Geometry check sheet. Reference: the model listing, model coordinates, mm. Face numbers are marked on the shaded views. A direction names the side the tool comes from. Give positions to 0.01 mm unless a question says otherwise; leave off trailing zeros. Loops run counter-clockwise (first coordinate to the right, second up) from the corner with the lowest first, then second, coordinate; pieces in that order, holes last. Notation, with made-up numbers: (-4.5, 50.25) -> (40.5, 50.25) arc R16 ccw to (40.5, 56.25) -> close; hole circle Ø2 at (-16, -13.5). An arc over 180 degrees is marked (long way). One line per question, with ' | ' between items.
from build123d import *

# Parameters (mm, degrees)
F0_W     = 80
F0_H     = 40
F1_DEPTH = 5
F2_W     = 66
F2_H     = 28
F2_W_2   = 60
F2_H_2   = 22
F3_DEPTH = 15
F4_R     = 2
F5_SIZE  = 1


with BuildPart() as f1:
    # F0 (on Top) → F1 (new body)
    with BuildSketch(Plane.XY):
        Rectangle(F0_W, F0_H)
    extrude(amount=F1_DEPTH)

    # F2 (on face) → F3 (join)
    with BuildSketch(Plane.XY.offset(5)):
        Rectangle(F2_W, F2_H)
        Rectangle(F2_W_2, F2_H_2, mode=Mode.SUBTRACT)
    extrude(amount=F3_DEPTH)

    # F4
    f4_edges = [f1.edges().sort_by_distance(p)[0] for p in [
        (0, -20, 0),
        (-40, 0, 0),
        (0, 20, 0),
        (40, 0, 0),
    ]]
    fillet(f4_edges, radius=F4_R)

    # F5
    f5_edges = [f1.edges().sort_by_distance(p)[0] for p in [
        (-33, -14, 12.5),
        (-33, 14, 12.5),
        (33, -14, 12.5),
        (33, 14, 12.5),
    ]]
    chamfer(f5_edges, length=F5_SIZE)


solid = f1.part
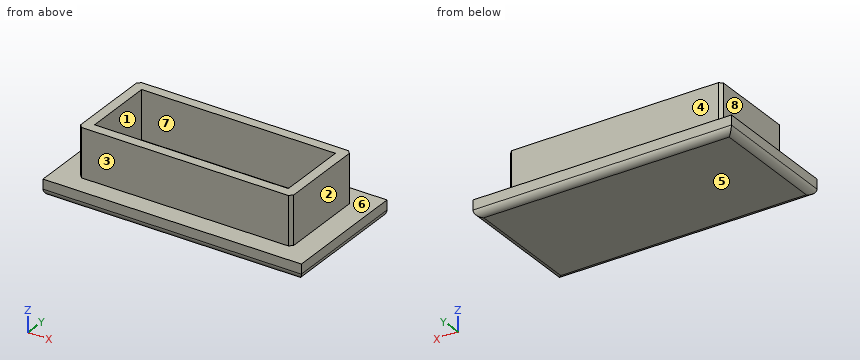
Item 1: Sectioned sample at B-B (y = 0). Record the cut outline in (x, z).
Result:
outline: (-40, 2) arc R2 ccw to (-38, 0) -> (38, 0) arc R2 ccw to (40, 2) -> (40, 5) -> (33, 5) -> (33, 20) -> (30, 20) -> (30, 5) -> (-30, 5) -> (-30, 20) -> (-33, 20) -> (-33, 5) -> (-40, 5) -> close
Item 2: Sectioned sample at C-C (x = -8.5). Record the cut outline in (y, z).
Result:
outline: (-20, 2) arc R2 ccw to (-18, 0) -> (18, 0) arc R2 ccw to (20, 2) -> (20, 5) -> (14, 5) -> (14, 20) -> (11, 20) -> (11, 5) -> (-11, 5) -> (-11, 20) -> (-14, 20) -> (-14, 5) -> (-20, 5) -> close
Item 3: Set-up check for the marked faces 1, 2, 3, 4 and 5: record each of +Z, -Z, +X, -X, +Y, -Y from which the full face is reachable in a straight line by a thin tool's end or side.
Result:
face 1: +Z | face 2: +Z, +X, +Y, -Y | face 3: +Z, +X, -X, -Y | face 4: +Z, +X, -X, +Y | face 5: -Z, +X, -X, +Y, -Y
Item 4: Sectioned sample at D-D (x = 31). Record the cut outline in (y, z).
Result:
outline: (-20, 2) arc R2 ccw to (-18, 0) -> (18, 0) arc R2 ccw to (20, 2) -> (20, 5) -> (14, 5) -> (14, 20) -> (-14, 20) -> (-14, 5) -> (-20, 5) -> close
Item 5: Sectioned sample at A-A (z = 14.5). Record the cut outline in (x, y), plus the area to 3 significant figures.
Result:
outline: (-33, -13) -> (-32, -14) -> (32, -14) -> (33, -13) -> (33, 13) -> (32, 14) -> (-32, 14) -> (-33, 13) -> close; hole (-30, -11) -> (30, -11) -> (30, 11) -> (-30, 11) -> close | area: 526 mm2
Item 6: Depth check by flat-ended pin: pin 1 Ø7.5 at (x, z) = (-15, 12.5) entering from +Y; pin 2 Ø6.5 at (x, y) = (-13.5, -0.5) entering from +Z; pin 3 Ø4.5 at (y, z) = (0, 10.5) entering from +X; pin 4 Ø10 at (y, z) = (-6, 8.5) entering from +X. Enter the tip coordinate at first touch or a pass-through.
Result:
pin 1: y = 14 | pin 2: z = 5 | pin 3: x = 33 | pin 4: x = 40
Item 7: Scan lines: probe 1 along Y at (x, z) = (17, 14); probe 2 along X at (y, z) = (7.5, 12.75); probe 3 along Z at (x, y) = (-28.5, 10.5). Record each from-to range of solid material in increasing order.
Result:
probe 1: -14 to -11, 11 to 14 | probe 2: -33 to -30, 30 to 33 | probe 3: 0 to 5
Item 8: Release check for a two-part mould opening along X. For the marked faces 6, 7 and 8 record: pulls with the +X half, pulls with the -X half, needs draft (parallel to the pull), parting line crosses it, or undercut.
Result:
face 6: needs draft | face 7: undercut | face 8: pulls with the -X half
